Read the model definition and answer for the solid it produces. Units are mm, in the model's axes. A direction names the side the tool comes from. Round coordinates to 2 decimals unless told otherwise and drop trailing zeros. Order: outer loops, then holes, each group sorted by start corner. A loop starts at its lowest first (then second) coordinate and runs counter-clockwise, first axis right, second up. Notation, with made-up numbers: (59, 2.5) - (88, 2.5) arc R13 cw to (88, 8.5) - close; hole circle Ø6 at (66, 54.5). An arc over 180 degrees is marked (long way). Answer as a JSON object with one key per item and string values. Group by question number.
Q1. A cutting plane is placed at A-A on x = 14. Determine the outline of the cut face in (y, z) (3 decimals).
Q2. Consider line 1 (X direction, y = -2134.5, z = 47) (3 decimals); line 2 (Z direction, x = 41, y = -1138) (3 decimals); line 3 (Y direction, x = 48, z = 56). Determine where each line is inside the solid, lowest interval first.
Q3. A cutting plane is placed at C-C on z = 33.5. Determine the outline of the cut face in (x, y) (3 decimals), and give its area (3 significant figures).
Q4. Given pin 1 Ø8 at (x, z) = (40, 50) entering from -Y; pin 2 Ø12 at (x, z) = (8.5, 43.5) entering from -Y, each flat-ended and moving along its own axis, determine where each tip first touches the part or whether it passes through.
Q5. A cutting plane is placed at B-B on y = -361. Determine the outline of the cut face in (x, z) (3 decimals), and give its area (3 significant figures).
Q6. The mould has two halves that part along Z. Classify faces 1 (the flat face through (25, -1202, 98.425)), 2 (the flat face through (25, -1202, 101.6)), 3 (the flat face through (3, -3, 51)), 4 (the flat face through (47.625, -1203, 50)): pulls with the +Z half, pulls with the -Z half, needs draft (parallel to the pull), parting line crosses it, or undercut.
Q7. A tool of negligible diameter and unlimited length cuts with its end or side. For faces 5 (the flat face through (3.175, -1202, 50)), 6 (the flat face through (0, -1202, 50)), from which of +Z, -Z, +X, -X, +Y, -Y can it reach the whole face along a straight path? Write none if from no direction.
```python
from build123d import *

# Parameters (mm, degrees)
F0_W     = 50.8
F0_H     = 101.6
F0_W_2   = 44.45
F0_H_2   = 95.25
F1_DEPTH = 2438.4
F3_DEPTH = 135.382
F4_R     = 5.08


with BuildPart() as f1:
    # F0 (on Front) → F1 (new body)
    with BuildSketch(Plane.XZ):
        with Locations((25.4, 50.8)):
            Rectangle(F0_W, F0_H)
        with Locations((25.4, 50.8)):
            Rectangle(F0_W_2, F0_H_2, mode=Mode.SUBTRACT)
    extrude(amount=F1_DEPTH)

    # F2 (on face) → F3 (cut)
    with BuildSketch(Plane.XY.offset(101.6)):
        Polygon((50.8, 0), (0, 0), (50.8, -50.8), align=None)
        Polygon((50.8, -2387.6), (0, -2438.4), (50.8, -2438.4), align=None)
    extrude(amount=-F3_DEPTH, mode=Mode.SUBTRACT)

    # F4
    f4_edges = [f1.edges().sort_by_distance(p)[0] for p in [
        (50.8, -1219.2, 101.6),
        (0, -1219.2, 101.6),
        (50.8, -1219.2, 0),
        (0, -1219.2, 0),
    ]]
    fillet(f4_edges, radius=F4_R)


solid = f1.part
```
Result set:
{
 "1": {"outline": "(-2424.4, 0) - (-14, 0) - (-14, 3.175) - (-2424.4, 3.175) - close; (-2424.4, 98.425) - (-14, 98.425) - (-14, 101.6) - (-2424.4, 101.6) - close"},
 "2": {"line 1": "x = 0 to 3.175, 47.625 to 50.8", "line 2": "z = 0 to 3.175, 98.425 to 101.6", "line 3": "y = -2390.4 to -48"},
 "3": {"outline": "(0, -2438.4) - (3.175, -2435.225) - (3.175, -3.175) - (0, 0) - close; (47.625, -2390.775) - (50.8, -2387.6) - (50.8, -50.8) - (47.625, -47.625) - close", "area": "15,200 mm²"},
 "4": {"pin 1": "passes through", "pin 2": "stops at y = -2435.9"},
 "5": {"outline": "(0, 5.08) arc R5.08 ccw to (5.08, 0) - (45.72, 0) arc R5.08 ccw to (50.8, 5.08) - (50.8, 96.52) arc R5.08 ccw to (45.72, 101.6) - (5.08, 101.6) arc R5.08 ccw to (0, 96.52) - close; hole (3.175, 3.175) - (47.625, 3.175) - (47.625, 98.425) - (3.175, 98.425) - close", "area": "905 mm²"},
 "6": {"face 1": "undercut", "face 2": "pulls with the +Z half", "face 3": "needs draft", "face 4": "undercut"},
 "7": {"face 5": "+Y, -Y", "face 6": "+Z, -Z, -X, +Y, -Y"}
}
